Can you work these out from the model? Positions are in its coordinate system, mm. Face numbers are marked on the shaded views. A direction names the side the tool comes from. Coordinates: 2 decimals unless noted, no trailing zeros. Order: outer loops, then holes, each group sorted by start corner. A loop starts at its lowest first (then second) coordinate and runs counter-clockwise, first axis right, second up. Notation, with made-up numbers: (69.5, 55.25) - (74.5, 55.25) arc R14 cw to (74.5, 60.25) - close; hole circle Ø11 at (-32, -16.5). An arc over 180 degrees is marked (long way). Return JSON: item names as keys, results as strings. Group by question number.
1) If I drill on line 1 along X through (y, z) = (328.75, 27.5); line 2 along X through (y, z) = (329.75, -16); line 3 along X through (y, z) = (332, 7.5), over which ranges is the centre line in solid material (lowest first)?
2) For pin 1 Ø4.5 at (x, y) = (9, 327) entering from -Z; pin 2 Ø1 at (y, z) = (326.5, -2.5) entering from +X; pin 3 Ø4 at (x, y) = (11, 336.5) entering from +Z, each with a flat end and sliding along its axis, tell me the tip position at first contact or that it passes through.
3) If we mould it in two halves opening along Z, with no side actions, what happens to the marked faces 1, 2, 3 and 4? For each: pulls with the +Z half, pulls with the -Z half, needs draft (parallel to the pull), parting line crosses it, or undercut.
4) Imagine slicing it at B-B (z = 49). Write out the boundary of the cut face in (x, y), and give its area (3 significant figures).
5) Which directions (+Z, -Z, +X, -X, +Y, -Y) give clear straight access to the entire face, cutting with the end or side of a thin tool? Please do the marked faces 5, 6 and 7.
6) Imagine slicing it at A-A (x = 15). Write out the boundary of the cut face in (y, z), and give its area (3 significant figures).
7) Imagine slicing it at C-C (y = 342.5). Write out the boundary of the cut face in (x, z).
8) Imagine slicing it at D-D (x = -3). Write out the boundary of the cut face in (y, z), and give its area (3 significant figures).
Autodesk Inventor part; units mm, degrees
ref_plane "Work Plane1" through (0, 0, 0) normal (0, 0, 1) x (1, 0, 0)
ref_plane "Work Plane2" through (0, 0, 0) normal (0, 0, 1) x (1, 0, 0)
ref_plane "YZ Plane" through (0, 0, 0) normal (1, 0, 0) x (0, 1, 0)
ref_plane "Work Plane1" through (0, 0, 0) normal (0, 0, 1) x (1, 0, 0)
ref_plane "Work Plane2" through (0, 0, 0) normal (0, 0, 1) x (1, 0, 0)
sketch "Sketch2" plane through (0, 0, 0) normal (0, 0, 1) x (1, 0, 0)
  line L0 (0, 0) -> (19.05, 0)
  line L1 (19.05, 0) -> (19.05, 431.8) construction
  line L2 (0, 431.8) -> (19.05, 431.8)
  line L3 (0, 0) -> (0, 431.8) construction
  line L4 (18.5, 323.6774) -> (1.5, 323.6774)
  line L5 (18.5, 323.6774) -> (19.1476, 323.6774)
  line L6 (1.5, 323.6774) -> (0, 323.6774)
  line L7 (-4.8174, 323.6774) -> (23.8674, 323.6774)
  line L8 (23.8674, 323.6774) -> (23.8674, 332.1879)
  line L9 (23.8674, 332.1879) -> (-4.8174, 332.1879)
  line L10 (-4.8174, 332.1879) -> (-4.8174, 323.6774)
  line L11 (9.525, 431.8) -> (9.525, 312.4258) construction
  line L12 (9.525, 327.9326) -> (-4.8174, 327.9326) construction
  line L13 (23.8674, 327.9326) -> (9.525, 327.9326) construction
extrude "Extrusion1" add sketch "Sketch2" along normal blind 61.9125
sketch "Sketch3" plane through (-4.8174, 323.6774, 0) normal (0, -1, 0) x (1, 0, 0)
  arc A0 (8.4674, 58.3733) -> (11.1674, 58.3733) centre (9.8174, 56.7) ccw
  arc A1 (18.4674, 58.3733) -> (21.1674, 58.3733) centre (19.8174, 56.7) ccw
  arc A2 (11.1674, 7.0267) -> (8.4674, 7.0267) centre (9.8174, 8.7) ccw
  arc A3 (21.1674, 7.0267) -> (18.4674, 7.0267) centre (19.8174, 8.7) ccw
  circle A4 centre (9.8174, 8.7) radius 2.15
  circle A5 centre (19.8174, 8.7) radius 2.15
  circle A6 centre (9.8174, 56.7) radius 2.15
  circle A7 centre (19.8174, 56.7) radius 2.15
  point P0 (4.8174, 0)
extrude "Extrusion2" cut sketch "Sketch3" against normal through all
sketch "Sketch4" plane through (-4.8174, 332.1879, 0) normal (0, 1, 0) x (1, 0, 0)
  line L0 (4.8174, -14.2) -> (4.8174, -51.2)
  line L1 (6.3174, -52.7) -> (23.3174, -52.7)
  line L2 (24.8174, -51.2) -> (24.8174, -14.2)
  line L3 (23.3174, -12.7) -> (6.3174, -12.7)
  line L4 (4.8174, -52.7) -> (24.8174, -52.7)
  line L5 (24.8174, -52.7) -> (24.8174, -12.7)
  line L6 (24.8174, -12.7) -> (4.8174, -12.7)
  line L7 (4.8174, -12.7) -> (4.8174, -52.7)
  point P0 (4.8174, 0)
extrude "Extrusion3" cut sketch "Sketch4" against normal through all
sketch "Sketch6" plane through (0, 0, 0) normal (0, 0, -1) x (-1, 0, 0)
  line L0 (4.8174, 323.6774) -> (-23.8674, 323.6774)
  line L1 (4.8174, 332.1879) -> (4.8174, 323.6774)
  line L2 (-23.8674, 332.1879) -> (4.8174, 332.1879)
  line L3 (-23.8674, 323.6774) -> (-23.8674, 332.1879)
  point P0 (0, 0)
extrude "Extrusion4" add sketch "Sketch6" along normal blind 19.05
sketch "Sketch7" plane through (-4.8174, 332.1879, 61.9125) normal (0, 1, 0) x (1, 0, 0)
  line L0 (4.8174, 70.6755) -> (4.8174, 80.9625)
  line L1 (4.8174, 61.9125) -> (4.8174, 70.6755)
  line L2 (23.8674, 61.9125) -> (23.8674, 70.6755)
  line L3 (23.8674, 71.4375) -> (23.8674, 80.9625)
  line L4 (23.8674, 61.9125) -> (4.8174, 61.9125)
  line L5 (4.8174, 61.9125) -> (4.8174, 80.9625)
  line L6 (4.8174, 80.9625) -> (23.8674, 80.9625)
  line L7 (23.8674, 80.9625) -> (23.8674, 61.9125)
extrude "Extrusion5" cut sketch "Sketch7" against normal through all
sketch "Sketch8" plane through (-4.8174, 332.1879, 61.9125) normal (0, 1, 0) x (1, 0, 0)
  line L0 (28.6847, 80.9625) -> (28.6847, 0)
  line L1 (0, 80.9625) -> (0, 0)
  line L2 (4.8174, 61.9125) -> (4.8174, 80.9625)
  line L3 (0, 80.9625) -> (4.8174, 80.9625)
  line L4 (0, 80.9625) -> (0, 0)
  line L5 (28.6847, 0) -> (0, 0)
  line L6 (28.6847, 80.9625) -> (28.6847, 0)
  line L7 (23.8674, 80.9625) -> (28.6847, 80.9625)
  line L8 (23.8674, 80.9625) -> (23.8674, 61.9125)
  line L9 (23.8674, 61.9125) -> (4.8174, 61.9125)
  line L10 (24.8174, 49.2125) -> (24.8174, 9.2125)
  line L11 (24.8174, 9.2125) -> (4.8174, 9.2125)
  line L12 (4.8174, 9.2125) -> (4.8174, 49.2125)
  line L13 (4.8174, 49.2125) -> (24.8174, 49.2125)
  circle A0 centre (9.8174, 5.2125) radius 2.15
  circle A1 centre (9.8174, 53.2125) radius 2.15
  circle A2 centre (19.8174, 53.2125) radius 2.15
  circle A3 centre (19.8174, 5.2125) radius 2.15
  line L14 (28.6847, 56.7746) -> (0, 56.7746)
  line L15 (28.6847, 56.7746) -> (57.3695, 56.7746) construction
  point P0 (4.8174, 61.9125)
  dimension "d10" = 180
extrude "Extrusion6" add sketch "Sketch8" along normal blind 12.7 contours L0 L14 L1 L3 L2 L9 L8 L7
sketch "Sketch10" plane through (23.8674, 323.6774, 61.9125) normal (1, 0, 0) x (0, 0, -1)
  point P0 (61.9125, -323.6774)
sketch "Sketch11" plane through (-4.8174, 323.6774, 61.9125) normal (-1, 0, 0) x (0, 0, 1)
  line L0 (0, 0) -> (-80.9625, 0)
  line L1 (0, 8.5105) -> (0, 0)
  line L2 (-56.7746, 8.5105) -> (0, 8.5105)
  line L3 (-56.7746, 8.5105) -> (-56.7746, 21.2105)
  line L4 (-80.9625, 21.2105) -> (-56.7746, 21.2105)
  line L5 (-80.9625, 0) -> (-80.9625, 21.2105)
  circle A0 centre (-66.9806, 14.1192) radius 1.7859
  circle A1 centre (-70.7565, 7.0913) radius 1.7859
  line L6 (-66.9806, 14.1192) -> (-66.9806, 21.2105) construction
  line L7 (-70.7565, 7.0913) -> (-70.7565, 0) construction
  line L8 (-80.9625, 0) -> (0, 0) construction
  line L9 (-70.7565, 7.0913) -> (-80.9625, 7.0913) construction
  line L10 (-80.9625, 0) -> (-80.9625, 21.2105) construction
  line L11 (-66.9806, 14.1192) -> (-56.7746, 14.1192) construction
  point P0 (-61.9125, -323.6774)
  dimension "d13" = 3.5719
  dimension "d14" = 3.5719
extrude "Extrusion7" cut sketch "Sketch11" against normal through all contours A0 | A1
chamfer "Chamfer1" distance 4.7625 angle 45 2 edges at (23.8674, 323.6774, 21.4312) (-4.8174, 323.6774, 21.4312)
properties part number "servo mount"
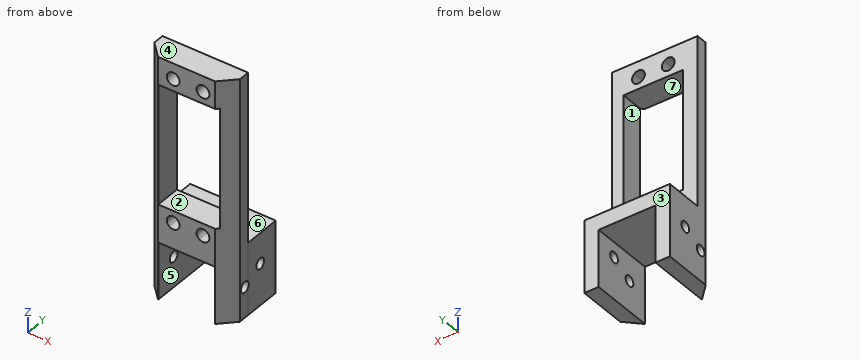
Calculated:
{
 "1": {"line 1": "-4.82 to 0, 20 to 23.87", "line 2": "-4.82 to 0, 19.05 to 23.87", "line 3": "-4.82 to 3.22, 6.78 to 13.22, 16.78 to 23.87"},
 "2": {"pin 1": "z = 0", "pin 2": "x = 22.43", "pin 3": "z = 5.14"},
 "3": {"face 1": "undercut", "face 2": "undercut", "face 3": "needs draft", "face 4": "pulls with the +Z half"},
 "4": {"outline": "(-4.82, 328.44) - (-0.05, 323.68) - (0, 323.68) - (0, 332.19) - (-4.82, 332.19) - close; (20, 324.57) - (23.87, 328.44) - (23.87, 332.19) - (20, 332.19) - close", "area": "51.6 mm2"},
 "5": {"face 5": "-Z, +Y, -Y", "face 6": "+Z, +X, -X, +Y", "face 7": "+Y, -Y"},
 "6": {"outline": "(323.68, 0) - (344.89, 0) - (344.89, 5.14) - (332.19, 5.14) - (332.19, 6.55) - (323.68, 6.55) - close; (323.68, 10.85) - (332.19, 10.85) - (332.19, 12.7) - (323.68, 12.7) - close; (323.68, 52.7) - (332.19, 52.7) - (332.19, 54.55) - (323.68, 54.55) - close; (323.68, 58.85) - (332.19, 58.85) - (332.19, 61.91) - (323.68, 61.91) - close", "area": "179 mm2"},
 "7": {"outline": "(-4.82, -19.05) - (0, -19.05) - (0, 0) - (19.05, 0) - (19.05, -19.05) - (23.87, -19.05) - (23.87, 5.14) - (-4.82, 5.14) - close"},
 "8": {"outline": "(326.62, -19.05) - (344.89, -19.05) - (344.89, 5.14) - (332.19, 5.14) - (332.19, 61.91) - (326.62, 61.91) - close; hole circle Ø3.57 at (330.77, -8.84); hole circle Ø3.57 at (337.8, -5.07)", "area": "738 mm2"}
}
